Autodesk Inventor part; units mm, degrees
ref_plane "YZ Plane" through (0, 0, 0) normal (1, 0, 0) x (0, 1, 0)
ref_plane "XZ Plane" through (0, 0, 0) normal (0, 1, 0) x (-1, 0, 0)
ref_plane "XY Plane" through (0, 0, 0) normal (0, 0, 1) x (1, 0, 0)
sketch "Sketch1" plane through (0, 0, 0) normal (0, 1, 0) x (-1, 0, 0)
  circle A0 centre (0, 0) radius 22.1996
  dimension "d0" = 44.3992
extrude "Extrusion1" add sketch "Sketch1" along normal blind 305.1302
sketch "Sketch2" plane through (0, 305.1302, 0) normal (0, 1, 0) x (1, 0, 0)
  circle A0 centre (0, 0) radius 14.4526
  circle A1 centre (0, 0) radius 12.6365
  dimension "d3" = 28.9052
  dimension "d4" = 25.273
extrude "Extrusion2" cut sketch "Sketch2" against normal blind 1.8034
sketch "Sketch3" plane through (0, 305.1302, 0) normal (0, 1, 0) x (1, 0, 0)
  circle A0 centre (0, 0) radius 10.9441
  circle A1 centre (0, 0) radius 12.6365
  dimension "d7" = 1.6924
extrude "Extrusion3" cut sketch "Sketch3" against normal blind 14.6558 draft -17 contours A0
sketch "Sketch5" plane through (0, 290.4744, 0) normal (0, 1, 0) x (1, 0, 0)
  circle A0 centre (0, 0) radius 6.4634
extrude "Extrusion4" cut sketch "Sketch5" against normal blind 355.6
sketch "Sketch6" plane through (0, 0, 0) normal (0, -1, 0) x (1, 0, 0)
  circle A0 centre (0, 0) radius 19.05
  circle A1 centre (0, 0) radius 22.1996
  dimension "d13" = 38.1
  dimension "d14" = 44.3992
extrude "Extrusion5" cut sketch "Sketch6" against normal blind 290.449 contours A0
sketch "Sketch7" plane through (0, 0, 0) normal (0, -1, 0) x (1, 0, 0)
  circle A0 centre (0, 0) radius 22.1996
extrude "Extrusion6" cut sketch "Sketch7" against normal blind 167.3352
sketch "Sketch8" plane through (0, 305.1302, 0) normal (0, 1, 0) x (1, 0, 0)
  point P0 (0, 0)
  point P1 (18.415, 0)
  point P2 (9.2075, 15.9479)
  point P3 (-9.2075, 15.9479)
  point P4 (-18.415, 0)
  point P5 (-9.2075, -15.9479)
  point P6 (9.2075, -15.9479)
  dimension "d19" = 18.415
  dimension "d22" = 360
properties part number "LED holder Thing"
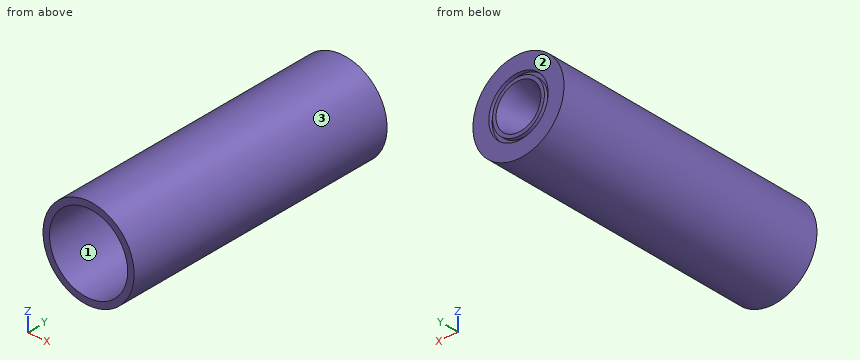
Could you check a few things on this model? Use its own coordinates, in mm. Face numbers are marked on the shaded views. Round coordinates to 2 decimals unless told otherwise and drop trailing zeros. Loops run counter-clockwise (first coordinate to the right, second up) from the corner with the lowest first, then second, coordinate; pieces in that order, holes last. Notation, with made-up numbers: (-4.5, 67) -> (8.5, 67) arc R14 ccw to (8.5, 84) -> close; hole circle Ø2 at (-14.75, 50.25). An arc over 180 degrees is marked (long way). Use CSV: the item, a comma, the result in double quotes.
(1) If we mould it in two halves opening along Z, with no side actions, what happens to the marked faces 1, 2 and 3? For each: +Z half, -Z half, draft (parallel to the pull), parting line (faces both ways), or undercut.
Return value:
face 1,"undercut"
face 2,"draft"
face 3,"parting line"
(2) If I drill on probe 1 along Z at (x, y) = (0, 304.25) (1 decimal); probe 2 along Z at (x, y) = (0, 204); probe 3 along Z at (x, y) = (0, 304.7), over which ranges is the centre line in solid material (lowest first)? Write a range as [from, to].
Return value:
probe 1,"z = [-22.2, -14.5], [-12.6, -10.7], [10.7, 12.6], [14.5, 22.2]"
probe 2,"z = [-22.2, -19.05], [19.05, 22.2]"
probe 3,"z = [-22.2, -14.45], [-12.64, -10.81], [10.81, 12.64], [14.45, 22.2]"
(3) Will these pins go through, and if not, where does the flat tip stop? pin 1 Ø12 at (x, z) = (7.5, -8.5) entering from -Y; pin 2 Ø5 at (x, y) = (-6.5, 208) entering from -Z; pin 3 Ø1 at (y, z) = (235.5, 16) entering from -X; pin 4 Ø1 at (y, z) = (258.5, 0.5) entering from -X.
Return value:
pin 1,"stops at y = 290.45"
pin 2,"stops at z = -21.84"
pin 3,"stops at x = -15.89"
pin 4,"stops at x = -22.2"
(4) Suppose I cut it at D-D on z = 17.5. Write out the boundary of the cut face in (x, y).
Return value:
outline,"(-13.66, 167.34) -> (-7.53, 167.34) -> (-7.53, 290.45) -> (7.53, 290.45) -> (7.53, 167.34) -> (13.66, 167.34) -> (13.66, 305.13) -> (-13.66, 305.13) -> close"
(5) Suppose I cut it at B-B on y = 203. Write out the boundary of the cut face in (x, z).
Return value:
outline,"circle Ø44.4 at (0, 0); hole circle Ø38.1 at (0, 0)"
